Autodesk Inventor part; units mm, degrees
ref_plane "YZ Plane" through (0, 0, 0) normal (1, 0, 0) x (0, 1, 0)
ref_plane "XZ Plane" through (0, 0, 0) normal (0, 1, 0) x (-1, 0, 0)
ref_plane "XY Plane" through (0, 0, 0) normal (0, 0, 1) x (1, 0, 0)
sketch "Sketch1" plane through (0, 0, 0) normal (0, 0, 1) x (1, 0, 0)
  line L0 (-35, 0) -> (35, 0) construction
  circle A0 centre (-35, 0) radius 16.05
  circle A1 centre (35, 0) radius 16.05
  arc A2 (-20, -20) -> (-50, -20) centre (-35, 0) ccw
  arc A3 (50, -20) -> (20, -20) centre (35, 0) ccw
  line L1 (-35, 25) -> (35, 25)
  line L2 (-50, -20) -> (50, -20)
  point P0 (0, 0)
  point P1 (0, 0)
  dimension "d0" = 70
  dimension "d1" = 32.1
  dimension "d3" = 50
  dimension "d38" = 20
extrude "Extrusion1" add sketch "Sketch1" along normal mid plane 48
fillet "Fillet3" radius 20 2 edges at (50, -20, 0) (-50, -20, 0)
sketch "Sketch10" plane through (-35, 25, 24) normal (0, 1, 0) x (1, 0, 0)
  line L0 (0, 48) -> (0, 0)
  line L1 (70, 0) -> (0, 0)
  line L2 (70, 48) -> (70, 0)
  line L3 (0, 48) -> (70, 48)
  point P0 (35, 24)
extrude "Extrusion4" add sketch "Sketch10" along normal blind 9
sketch "Sketch11" plane through (-35, 34, 24) normal (0, 1, 0) x (1, 0, 0)
  line L0 (19, 2.95) -> (51, 2.95)
  line L1 (51, 2.95) -> (51, 45.05)
  line L2 (51, 45.05) -> (19, 45.05)
  line L3 (19, 45.05) -> (19, 2.95)
  line L4 (19, 2.95) -> (51, 45.05) construction
  line L5 (51, 2.95) -> (19, 45.05) construction
  line L6 (0, 48) -> (0, 0)
  line L7 (0, 0) -> (70, 0)
  line L8 (70, 0) -> (70, 48)
  line L9 (70, 48) -> (0, 48)
  line L10 (27, 48) -> (43, 48)
  line L11 (43, 48) -> (43, 45.05)
  line L12 (43, 45.05) -> (27, 45.05)
  line L13 (27, 45.05) -> (27, 48)
  line L14 (27, 2.95) -> (27, 0)
  line L15 (35, 24) -> (35, 47.5578) construction
  line L16 (43, 2.95) -> (43, 0)
  point P0 (35, 45.05)
  point P1 (43, 0)
  point P2 (43, 2.95)
  dimension "d49" = 32
  dimension "d50" = 42.1
  dimension "d53" = 16
extrude "Extrusion5" cut sketch "Sketch11" against normal blind 12 contours L3 L2 L1 L0 | L0 L16 L7 L14 | L13 L9 L11 L2
sketch "Sketch12" plane through (-40, -20, -24) normal (0, -1, 0) x (1, 0, 0)
  line L0 (27.5, 14) -> (52.5, 14) construction
  line L1 (52.5, 14) -> (52.5, 34) construction
  line L2 (52.5, 34) -> (27.5, 34) construction
  line L3 (27.5, 34) -> (27.5, 14) construction
  line L4 (27.5, 14) -> (52.5, 34) construction
  line L5 (52.5, 14) -> (27.5, 34) construction
  point P0 (40, 24)
  dimension "d54" = 25
  dimension "d55" = 20
hole "Hole4" at (-12.5, -20, 10) at (12.5, -20, 10) at (12.5, -20, -10) at (-12.5, -20, -10) direction (0, 1, 0) diameter 3.2 end through all counterbore diameter 6.5 counterbore depth 20
fillet "Fillet4" radius 4 4 edges at (35, 29.5, 24) (35, 29.5, -24) (-35, 29.5, 24) (-35, 29.5, -24)
properties part number "Space Craft Braket" material "ABS Plastic"
Geometry: final body of the model. Coordinates: model frame, mm. A direction names the side the tool comes from. Give positions to 0.01 mm unless a question says otherwise; leave off trailing zeros. Order: outer loops, then holes, each group sorted by start corner. A loop starts at its lowest first (then second) coordinate and runs counter-clockwise, first axis right, second up. Notation, with made-up numbers: (-3, 87.25) -> (20, 87.25) arc R14 cw to (20, 93.25) -> close; hole circle Ø9 at (-9.5, 44). An arc over 180 degrees is marked (long way). Write each question's results on one line, items separated by ' | '. Start each with the question number.
1) Line query: line 1 (Z direction, x = -12.5, y = -8); line 2 (X direction, y = 10, z = 10); line 3 (X direction, y = -4, z = 16). Output: solid intervals per line, ascending. Write a range as from..to.
2) Section D-D (y = 27). Return loops of the section in (x, z).
3) Section B-B (x = -12.5). Return loops of the section in (y, z), then the cut area to 3 significant figures.
4) First-contact query: pin 1 (5 mm diameter, centred on x = -12.5, z = 10, fed in from -Y); pin 2 (6 mm diameter, centred on y = 18, z = -1, fed in from -X); pin 3 (8 mm diameter, centred on x = 43, y = 8, fed in from +Z); pin 4 (9.5 mm diameter, centred on y = 31, z = -3, fed in from -X). Flat tips, straight axial feed; report the tip coordinate or a pass-through.
5) Set-up query: faces 1 (the flat face through (11, 0, 9)), 2 (the flat face through (-16, 28, 0)), 3 (the flat face through (-35, 29, 0)), 4 (the flat face through (8, 28, 23)). Return all of +Z, -Z, +X, -X, +Y, -Y with unobstructed straight access to the full face (end or side cutting, diameter ignored); none if empty.
6) Section C-C (y = 7). Return loops of the section in (x, z).
7) Section A-A (z = -10). Count the separate pieces of the cut face and the enclosed holes in it, then the cut area to 3 significant figures.
8) Draft query along X for faces 5 (the flat face through (-1, -20, 0)), 6 (the flat face through (35, 29, 0)), 7 (the flat face through (-14, 0, -11)). Return one class per face: pulls with the +X half, pulls with the -X half, needs draft (parallel to the pull), parting line crosses it, or undercut.
Calculated:
1) line 1: -24..-13.25, -6.75..6.75, 13.25..24 | line 2: -57.91..-47.55, -22.45..-14.1, -10.9..10.9, 14.1..22.45, 47.55..57.91 | line 3: -59.6..-50.54, -19.46..19.46, 50.54..59.6
2) outline: (-35, -20) arc R4 ccw to (-31, -24) -> (-8, -24) -> (-8, -21.05) -> (-16, -21.05) -> (-16, 21.05) -> (-8, 21.05) -> (-8, 24) -> (-31, 24) arc R4 ccw to (-35, 20) -> close; (8, -24) -> (31, -24) arc R4 ccw to (35, -20) -> (35, 20) arc R4 ccw to (31, 24) -> (8, 24) -> (8, 21.05) -> (16, 21.05) -> (16, -21.05) -> (8, -21.05) -> close
3) outline: (-20, -24) -> (34, -24) -> (34, -21.05) -> (22, -21.05) -> (22, -11.6) -> (0, -11.6) -> (0, -13.25) -> (-20, -13.25) -> close; (-20, -6.75) -> (0, -6.75) -> (0, -8.4) -> (22, -8.4) -> (22, 8.4) -> (0, 8.4) -> (0, 6.75) -> (-20, 6.75) -> close; (-20, 13.25) -> (0, 13.25) -> (0, 11.6) -> (22, 11.6) -> (22, 21.05) -> (34, 21.05) -> (34, 24) -> (-20, 24) -> close | area: 1,690 mm2
4) pin 1: y = 0 | pin 2: x = -55 | pin 3: through | pin 4: x = -35
5) face 1: -Y | face 2: +Y | face 3: +Z, -Z, -X, +Y | face 4: +Z, -Z, +Y
6) outline: (-59, -24) -> (-49.44, -24) -> (-49.44, 24) -> (-59, 24) -> close; (-20.56, -24) -> (20.56, -24) -> (20.56, 24) -> (-20.56, 24) -> close; (49.44, -24) -> (59, -24) -> (59, 24) -> (49.44, 24) -> close; hole circle Ø3.2 at (-12.5, -10); hole circle Ø3.2 at (-12.5, 10); hole circle Ø3.2 at (12.5, -10); hole circle Ø3.2 at (12.5, 10)
7) separate pieces: 3 | enclosed holes: 2 | area: 3,190 mm2
8) face 5: needs draft | face 6: pulls with the +X half | face 7: undercut
